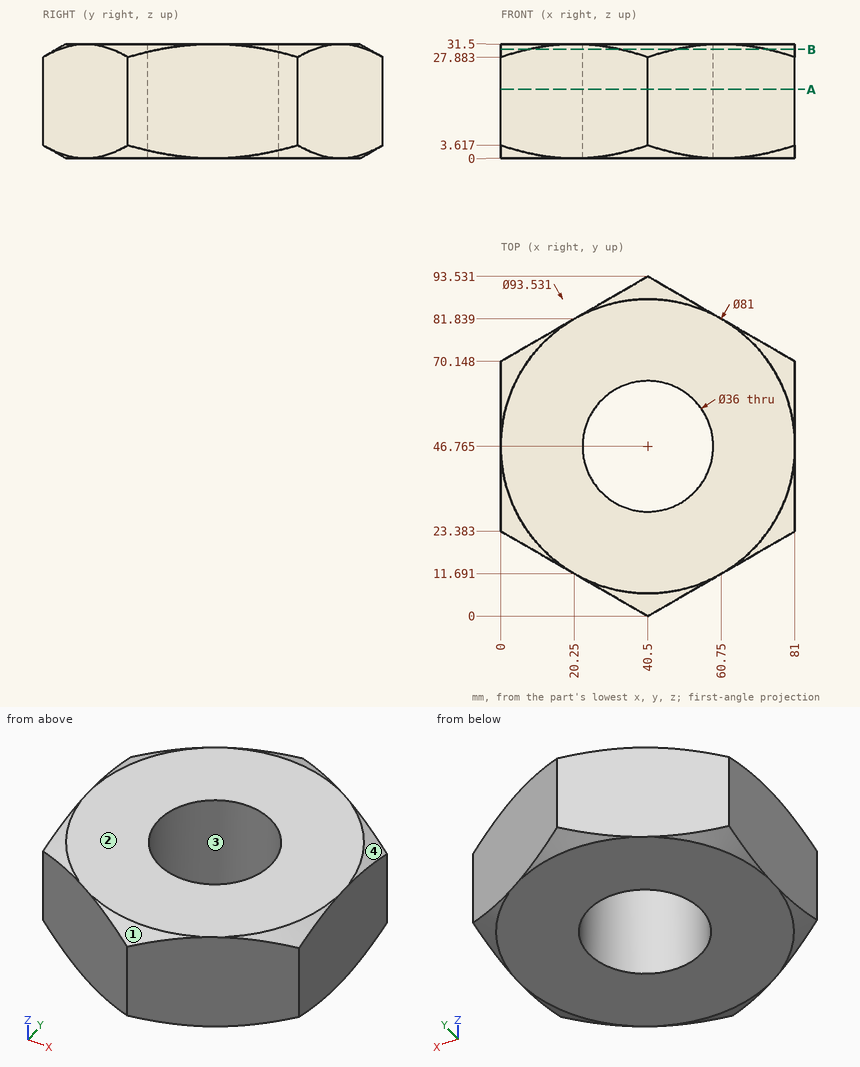
Study the drawing (mm; zero at the part's minimum x, y, z) and answer. Round coordinates to 2 decimals unless told otherwise and drop trailing zeros. Write each loop counter-clockwise with the first axis right and the second up, starting at its lowest first coordinate (ties: lowest second). Pieces come first, ordered by that corner, then holes.
1) Determine the mould class of the marked faces 1, 2, 3 and 4 for opening direction X: pulls with the +X half, pulls with the -X half, needs draft (parallel to the pull), parting line crosses it, or undercut.
2) A cutting plane is placed at A-A on z = 19. Determine the outline of the cut face in (x, y) (1 decimal), and give its area (3 significant figures).
3) A cutting plane is placed at B-B on z = 30. Determine the outline of the cut face in (x, y) (1 decimal).
4) Flat-ended cylindrical pins translate along their axes: P1, Ø3, axis at x = 26.5, y = 38.5, coming from the +Z side; P2, Ø1, axis at x = 47, z = 24, coming from the -Y side (1 decimal); P3, Ø10, axis at x = 54, z = 14, coming from the +Y side; P4, Ø1.5, axis at x = 31, z = 26, coming from the -Y side. Find the tip coordinate at first contact, or state that the pin passes through.
5) Consider probe 1 along Y at (x, z) = (40.5, 24) (1 decimal); probe 2 along Y at (x, z) = (34.5, 6.5) (1 decimal); probe 3 along X at (y, z) = (37, 9). Determine where each line is inside the solid, lowest interval first.
Entries:
1. face 1: parting line crosses it
1. face 2: needs draft
1. face 3: undercut
1. face 4: pulls with the +X half
2. outline: (0, 23.4) - (40.5, 0) - (81, 23.4) - (81, 70.1) - (40.5, 93.5) - (0, 70.1) - close; hole circle Ø36 at (40.5, 46.8)
2. area: 4,660 mm2
3. outline: (0, 32) arc R43.1 ccw to (7.5, 19.1) - (33, 4.3) arc R43.1 ccw to (48, 4.3) - (73.5, 19.1) arc R43.1 ccw to (81, 32) - (81, 61.5) arc R43.1 ccw to (73.5, 74.5) - (48, 89.2) arc R43.1 ccw to (33, 89.2) - (7.5, 74.5) arc R43.1 ccw to (0, 61.5) - close; hole circle Ø36 at (40.5, 46.8)
4. P1: passes through
4. P2: stops at y = 3.5
4. P3: stops at y = 88.62
4. P4: stops at y = 5.05
5. probe 1: y = 0 to 28.8, 64.8 to 93.5
5. probe 2: y = 3.5 to 29.8, 63.7 to 90.1
5. probe 3: x = 0 to 25.38, 55.62 to 81
